Can you work these out from the model? Positions are in its coordinate system, mm. A direction names the side the tool comes from. Round coordinates to 2 decimals unless told otherwise and drop trailing zeros. Order: outer loops, then holes, each group sorted by start corner. A loop starts at its lowest first (then second) coordinate and runs counter-clockwise, first axis right, second up. Notation, with made-up numbers: M -37,57.25 L 5,57.25 A11 ccw 5,75.25 Z; hole C -36,-10 d3. An arc over 180 degrees is marked long. Answer as a JSON object with one key per item and string values. Group by question number.
from build123d import *

# Parameters (mm, degrees)
SKETCH1_R                = 40
BOSS_EXTRUDE1_DEPTH      = 2
SKETCH4_R                = 3
BOSS_EXTRUDE3_DEPTH      = 2
FILLET2_R                = 4
CIRPATTERN2_COUNT        = 3
FILLET2_OF_CIRPATTERN2_R = 4
SKETCH5_R                = 10
CUT_EXTRUDE1_DEPTH       = 8
SKETCH6_R                = 2
CUT_EXTRUDE2_DEPTH       = 8
CIRPATTERN3_COUNT        = 3
CUT_EXTRUDE3_DEPTH       = 15
FILLET3_R                = 5
CIRPATTERN4_COUNT        = 3
FILLET3_OF_CIRPATTERN4_R = 5


with BuildPart() as part:
    # Sketch1 → Boss-Extrude1 (new body)
    with BuildSketch(Plane.XY):
        Circle(SKETCH1_R)
    extrude(amount=BOSS_EXTRUDE1_DEPTH)

    # Sketch4 → Boss-Extrude3 (add)
    with BuildSketch(Plane(origin=(0, 0, 0), x_dir=(-1, 0, 0), z_dir=(0, 0, -1))):
        with BuildLine():
            Line((-15.513007814, 36.869317712), (-18.669872981, 42.337168574))
            ThreePointArc((-18.669872981, 42.337168574), (-25.5, 44.167295593), (-27.330127019, 37.337168574))
            Line((-27.330127019, 37.337168574), (-24.173261852, 31.869317712))
            Line((-24.173261852, 31.869317712), (-15.513007814, 36.869317712))
        make_face()
        with Locations((-23, 39.837168574)):
            Circle(SKETCH4_R, mode=Mode.SUBTRACT)
    boss_extrude3 = extrude(amount=-BOSS_EXTRUDE3_DEPTH)

    # Fillet2
    fillet2_edges = [part.edges().sort_by_distance(p)[0] for p in [
        (15.513007814, 36.869317712, 1),
        (24.173261852, 31.869317712, 1),
    ]]
    fillet(fillet2_edges, radius=FILLET2_R)

    # CirPattern2: Boss-Extrude3 ×3 about axis
    cirpattern2_axis = Axis((0, 0, 0), (0, 0, 1))
    for i in range(1, CIRPATTERN2_COUNT):
        add(boss_extrude3.rotate(cirpattern2_axis, i * 360 / CIRPATTERN2_COUNT))

    # Fillet2 of CirPattern2
    fillet2_of_cirpattern2_edges = [part.edges().sort_by_distance(p)[0] for p in [
        (-39.686269666, -5, 1),
        (-39.686269666, 5, 1),
        (24.173261852, -31.869317712, 1),
        (15.513007814, -36.869317712, 1),
    ]]
    fillet(fillet2_of_cirpattern2_edges, radius=FILLET2_OF_CIRPATTERN2_R)

    # Sketch5 → Cut-Extrude1 (cut)
    with BuildSketch(Plane(origin=(0, 0, 0), x_dir=(-1, 0, 0), z_dir=(0, 0, -1))):
        Circle(SKETCH5_R)
    extrude(amount=-CUT_EXTRUDE1_DEPTH, mode=Mode.SUBTRACT)

    # Sketch6 → Cut-Extrude2 (cut)
    with BuildSketch(Plane(origin=(0, 0, 0), x_dir=(-1, 0, 0), z_dir=(0, 0, -1))):
        with Locations((-7, 12.124355653)):
            Circle(SKETCH6_R)
    cut_extrude2 = extrude(amount=-CUT_EXTRUDE2_DEPTH, mode=Mode.SUBTRACT)

    # CirPattern3: Cut-Extrude2 ×3 about axis
    cirpattern3_axis = Axis((0, 0, 0), (0, 0, 1))
    for i in range(1, CIRPATTERN3_COUNT):
        add(cut_extrude2.rotate(cirpattern3_axis, i * 360 / CIRPATTERN3_COUNT), mode=Mode.SUBTRACT)

    # Sketch7 → Cut-Extrude3 (cut)
    with BuildSketch(Plane(origin=(0, 0, 0), x_dir=(-1, 0, 0), z_dir=(0, 0, -1))):
        with BuildLine():
            ThreePointArc((-5.156603958, 19.323804895), (10, 17.320508076), (19.313207916, 5.196152423))
            Line((19.313207916, 5.196152423), (32.081926376, 5.196152423))
            ThreePointArc((32.081926376, 5.196152423), (16.25, 28.145825623), (-11.540963188, 30.381839455))
            Line((-11.540963188, 30.381839455), (-5.156603958, 19.323804895))
        make_face()
    cut_extrude3 = extrude(amount=-CUT_EXTRUDE3_DEPTH, mode=Mode.SUBTRACT)

    # Fillet3
    fillet3_edges = [part.edges().sort_by_distance(p)[0] for p in [
        (-32.081926376, 5.196152423, 1),
        (-19.313207916, 5.196152423, 1),
        (5.156603958, 19.323804895, 1),
        (11.540963188, 30.381839455, 1),
    ]]
    fillet(fillet3_edges, radius=FILLET3_R)

    # CirPattern4: Cut-Extrude3 ×3 about axis
    cirpattern4_axis = Axis((0, 0, 0), (0, 0, 1))
    for i in range(1, CIRPATTERN4_COUNT):
        add(cut_extrude3.rotate(cirpattern4_axis, i * 360 / CIRPATTERN4_COUNT), mode=Mode.SUBTRACT)

    # Fillet3 of CirPattern4
    fillet3_of_cirpattern4_edges = [part.edges().sort_by_distance(p)[0] for p in [
        (11.540963188, -30.381839455, 1),
        (5.156603958, -19.323804895, 1),
        (-19.313207916, -5.196152423, 1),
        (-32.081926376, -5.196152423, 1),
        (20.540963188, 25.185687033, 1),
        (14.156603958, 14.127652472, 1),
        (14.156603958, -14.127652472, 1),
        (20.540963188, -25.185687033, 1),
    ]]
    fillet(fillet3_of_cirpattern4_edges, radius=FILLET3_OF_CIRPATTERN4_R)


solid = part.part
Item 1: I'm going to push a flat-ended pin straight in: pin 1 Ø3.5 at (x, y) = (7, 12.12) entering from +Z. Where does the tip first touch, or does it pass through?
Item 2: On a 3-axis mill with a long thin cutter (end or side, diameter ignored), from which of +Z, -Z, +X, -X, +Y, -Y can I reach the whole of each face in a straight line? I mean faces 1 (the face through (-20.41, -34.4, 0.99)), 2 (the face through (7.601, 23.558, 0.986)), 3 (the face through (26.587, -36.051, 0.986)). Say none if no direction works.
Item 3: Suppose I cut it at D-D, the plane x = 30. Write out the boundary of the cut face in (y, z).
Item 4: If we mould it in two halves opening along X, with no side actions, what happens to faces 4 (the face through (-20.072, -6.023, 1.014)), 5 (the face through (-48.86, 0.9, 0.99)), 6 (the face through (25.374, 32.205, 1.014))? For each: +X half, -X half, draft (parallel to the pull), parting line (faces both ways), or undercut.
Item 5: Suppose I cut it at C-C, the plane y = 26. Write out the boundary of the cut face in (x, z), and give its area (3 significant figures).
Item 6: Suppose I cut it at B-B, the plane x = 0. Write out the boundary of the cut face in (y, z).
Item 7: Suppose I cut it at A-A, the plane y = 0. Write out the boundary of the cut face in (x, z), and give its area (3 significant figures).
Item 8: I need wall thicknesses on line 1 (Y direction, x = 7, z = 1.4); line 2 (Y direction, x = -17.5, z = 0.9); line 3 (X direction, y = -9, z = 1.5). Which ranges of each line are inside material? Lowest first, please.
Computed:
{
 "1": {"pin 1": "passes through"},
 "2": {"face 1": "+Z, -Z, -Y", "face 2": "+Z, -Z", "face 3": "+Z, -Z, +X"},
 "3": {"outline": "M -26.46,0 L -12.5,0 L -12.5,2 L -26.46,2 Z; M 12.5,0 L 26.46,0 L 26.46,2 L 12.5,2 Z"},
 "4": {"face 4": "undercut", "face 5": "undercut", "face 6": "+X half"},
 "5": {"outline": "M -30.4,0 L -19.5,0 L -19.5,2 L -30.4,2 Z; M 8.79,0 L 30.4,0 L 30.4,2 L 8.79,2 Z", "area": "65.0 mm^2"},
 "6": {"outline": "M -40,0 L -32.5,0 L -32.5,2 L -40,2 Z; M -20,0 L -10,0 L -10,2 L -20,2 Z; M 10,0 L 20,0 L 20,2 L 10,2 Z; M 32.5,0 L 40,0 L 40,2 L 32.5,2 Z"},
 "7": {"outline": "M -51,0 L -49,0 L -49,2 L -51,2 Z; M -43,0 L -16,0 L -16,2 L -43,2 Z; M -12,0 L -10,0 L -10,2 L -12,2 Z; M 10,0 L 20,0 L 20,2 L 10,2 Z; M 32.5,0 L 40,0 L 40,2 L 32.5,2 Z", "area": "97.0 mm^2"},
 "8": {"line 1": "y = -39.38 to -31.17, -22.52 to -14.12, -10.12 to -7.14, 7.14 to 10.12, 14.12 to 22.52, 31.17 to 39.38", "line 2": "y = -35.97 to -27.39, -9.68 to 9.68, 27.39 to 35.97", "line 3": "x = -38.97 to -30.39, -17.86 to -4.36, 4.36 to 17.86, 31.23 to 38.97"}
}
